from build123d import *

# Parameters (mm, degrees)
SKETCH_R          = 1.45
PAD001_DEPTH      = 1.6
SKETCH001_R       = 1.45
PAD002_DEPTH      = 16.25
POCKET_DEPTH      = 190.001
POCKET_DEPTH_BACK = 0.001
SKETCH003_R       = 1.45
PAD003_DEPTH      = 3.4
POCKET001_DEPTH   = 5
POCKET002_DEPTH   = 10
SKETCH031_R       = 1.125
PAD017_DEPTH      = 6
POCKET013_DEPTH   = 4
SKETCH033_R       = 3
POCKET014_DEPTH   = 5


with BuildPart() as part:
    # Sketch → Pad001 (new body)
    with BuildSketch(Plane.XY):
        with BuildLine():
            Line((12.25, 182), (190.25, 182))
            ThreePointArc((196.25, 176), (194.492641, 180.242641), (190.25, 182))
            Line((196.25, 176), (196.25, 3))
            ThreePointArc((190.25, -3), (194.492641, -1.242641), (196.25, 3))
            Line((190.25, -3), (12.25, -3))
            ThreePointArc((6.25, 3), (8.007359, -1.242641), (12.25, -3))
            Line((6.25, 3), (6.25, 97))
            Line((23.25, 97), (6.25, 97))
            ThreePointArc((23.25, 97), (28.906854, 99.343146), (31.25, 105))
            Line((31.25, 122), (31.25, 105))
            ThreePointArc((31.25, 122), (28.906854, 127.656854), (23.25, 130))
            Line((6.25, 130), (23.25, 130))
            Line((6.25, 130), (6.25, 176))
            ThreePointArc((12.25, 182), (8.007359, 180.242641), (6.25, 176))
        make_face()
        with Locations((11, 173.49762)):
            Circle(SKETCH_R, mode=Mode.SUBTRACT)
        with Locations((11, 89.49762)):
            Circle(SKETCH_R, mode=Mode.SUBTRACT)
        with Locations((180.742493, 173.605331)):
            Circle(SKETCH_R, mode=Mode.SUBTRACT)
        with Locations((181.761108, 91.056091)):
            Circle(SKETCH_R, mode=Mode.SUBTRACT)
        with Locations((44.67, 76.67)):
            Circle(SKETCH_R, mode=Mode.SUBTRACT)
        with Locations((44.67, 24.67)):
            Circle(SKETCH_R, mode=Mode.SUBTRACT)
        with Locations((191.67, 24.67)):
            Circle(SKETCH_R, mode=Mode.SUBTRACT)
        with Locations((191.67, 76.67)):
            Circle(SKETCH_R, mode=Mode.SUBTRACT)
        with BuildLine():
            ThreePointArc((40.25, 97.49762), (42.593146, 91.840766), (48.25, 89.49762))
            Line((168.624548, 89.49762), (48.25, 89.49762))
            ThreePointArc((168.624548, 89.49762), (174.281402, 91.840766), (176.624548, 97.49762))
            Line((176.624548, 122), (176.624548, 97.49762))
            ThreePointArc((176.624548, 122), (174.281402, 127.656854), (168.624548, 130))
            Line((48.25, 130), (168.624548, 130))
            ThreePointArc((48.25, 130), (42.593146, 127.656854), (40.25, 122))
            Line((40.25, 97.49762), (40.25, 122))
        make_face(mode=Mode.SUBTRACT)
        with BuildLine():
            ThreePointArc((15.25, 147), (17.593146, 141.343146), (23.25, 139))
            Line((168.563514, 139), (23.25, 139))
            ThreePointArc((168.563514, 139), (174.220369, 141.343146), (176.563514, 147))
            Line((176.563514, 165.49762), (176.563514, 147))
            ThreePointArc((176.563514, 165.49762), (174.220369, 171.154474), (168.563514, 173.49762))
            Line((23.25, 173.49762), (168.563514, 173.49762))
            ThreePointArc((23.25, 173.49762), (17.593146, 171.154474), (15.25, 165.49762))
            Line((15.25, 147), (15.25, 165.49762))
        make_face(mode=Mode.SUBTRACT)
        with BuildLine():
            ThreePointArc((51.67, 14), (54.013146, 8.343146), (59.67, 6))
            Line((176.67, 6), (59.67, 6))
            ThreePointArc((176.67, 6), (182.326854, 8.343146), (184.67, 14))
            Line((184.67, 68.67), (184.67, 14))
            ThreePointArc((184.67, 68.67), (182.326854, 74.326854), (176.67, 76.67))
            Line((59.67, 76.67), (176.67, 76.67))
            ThreePointArc((59.67, 76.67), (54.013146, 74.326854), (51.67, 68.67))
            Line((51.67, 14), (51.67, 68.67))
        make_face(mode=Mode.SUBTRACT)
    extrude(amount=-PAD001_DEPTH)

    # Sketch001 → Pad002 (join)
    with BuildSketch(Plane.XY):
        with BuildLine():
            ThreePointArc((51.67, 76.67), (44.67, 83.67), (37.67, 76.67))
            Line((37.67, 76.67), (37.67, 7))
            ThreePointArc((37.67, 7), (44.67, 0), (51.67, 7))
            Line((51.67, 7), (51.67, 76.67))
        make_face()
        with Locations((44.67, 76.67)):
            Circle(SKETCH001_R, mode=Mode.SUBTRACT)
        with Locations((44.67, 24.67)):
            Circle(SKETCH001_R, mode=Mode.SUBTRACT)
        with BuildLine():
            ThreePointArc((196.25, 76.67), (191.67, 81.25), (187.09, 76.67))
            Line((187.09, 76.67), (187.09, 4.58))
            ThreePointArc((187.09, 4.58), (191.67, 0), (196.25, 4.58))
            Line((196.25, 4.58), (196.25, 76.67))
        make_face()
        with Locations((191.67, 76.67)):
            Circle(SKETCH001_R, mode=Mode.SUBTRACT)
        with Locations((191.67, 24.67)):
            Circle(SKETCH001_R, mode=Mode.SUBTRACT)
    extrude(amount=PAD002_DEPTH)

    # Sketch002 (on Face56 of Pad002) → Pocket (cut, two sides)
    with BuildSketch(Plane.YZ.offset(196.25)) as pocket_sk:
        with BuildLine():
            ThreePointArc((31, 22), (28.87868, 21.12132), (28, 19))
            Line((28, 9), (28, 19))
            ThreePointArc((28, 9), (28.87868, 6.87868), (31, 6))
            Line((61, 6), (31, 6))
            ThreePointArc((61, 6), (63.12132, 6.87868), (64, 9))
            Line((64, 19), (64, 9))
            ThreePointArc((64, 19), (63.12132, 21.12132), (61, 22))
            Line((31, 22), (61, 22))
        make_face()
    extrude(amount=-POCKET_DEPTH, mode=Mode.SUBTRACT)
    extrude(pocket_sk.sketch, amount=POCKET_DEPTH_BACK, mode=Mode.SUBTRACT)

    # Sketch003 → Pad003 (join)
    with BuildSketch(Plane.XY.offset(-0.1)):
        with BuildLine():
            ThreePointArc((185.53296, 93.654078), (179.163121, 94.827943), (177.989256, 88.458104))
            Line((177.989256, 88.458104), (187.898148, 74.072013))
            ThreePointArc((187.898148, 74.072013), (194.267987, 72.898148), (195.441852, 79.267987))
            Line((195.441852, 79.267987), (185.53296, 93.654078))
        make_face()
        with Locations((191.67, 76.67)):
            Circle(SKETCH003_R, mode=Mode.SUBTRACT)
        with Locations((181.761108, 91.056091)):
            Circle(SKETCH003_R, mode=Mode.SUBTRACT)
        with BuildLine():
            ThreePointArc((12.691088, 93.936395), (6.561225, 91.188708), (9.308912, 85.058845))
            Line((9.308912, 85.058845), (42.978912, 72.231225))
            ThreePointArc((42.978912, 72.231225), (49.108775, 74.978912), (46.361088, 81.108775))
            Line((46.361088, 81.108775), (12.691088, 93.936395))
        make_face()
        with Locations((44.67, 76.67)):
            Circle(SKETCH003_R, mode=Mode.SUBTRACT)
        with Locations((11, 89.49762)):
            Circle(SKETCH003_R, mode=Mode.SUBTRACT)
        with BuildLine():
            ThreePointArc((15.25, 173.49762), (11, 177.74762), (6.75, 173.49762))
            Line((6.75, 173.49762), (6.75, 165.49762))
            ThreePointArc((6.75, 165.49762), (11, 161.24762), (15.25, 165.49762))
            Line((15.25, 165.49762), (15.25, 173.49762))
        make_face()
        with Locations((11, 173.49762)):
            Circle(SKETCH003_R, mode=Mode.SUBTRACT)
        with BuildLine():
            ThreePointArc((180.742493, 178.185331), (176.162493, 173.605331), (180.742493, 169.025331))
            Line((180.742493, 169.025331), (191.67, 169.025331))
            ThreePointArc((191.67, 169.025331), (196.25, 173.605331), (191.67, 178.185331))
            Line((191.67, 178.185331), (180.742493, 178.185331))
        make_face()
        with Locations((180.742493, 173.605331)):
            Circle(SKETCH003_R, mode=Mode.SUBTRACT)
    extrude(amount=PAD003_DEPTH)

    # Sketch004 → Pocket001 (cut)
    with BuildSketch(Plane.XY):
        with BuildLine():
            ThreePointArc((75.723694, 140.85524), (75.016587, 140.562347), (74.723694, 139.85524))
            Line((74.723694, 134.85524), (74.723694, 139.85524))
            ThreePointArc((74.723694, 134.85524), (75.016587, 134.148133), (75.723694, 133.85524))
            Line((91.423694, 133.85524), (75.723694, 133.85524))
            ThreePointArc((91.423694, 133.85524), (92.130801, 134.148133), (92.423694, 134.85524))
            Line((92.423694, 139.85524), (92.423694, 134.85524))
            ThreePointArc((92.423694, 139.85524), (92.130801, 140.562347), (91.423694, 140.85524))
            Line((75.723694, 140.85524), (91.423694, 140.85524))
        make_face()
        with BuildLine():
            ThreePointArc((129.923694, 140.85524), (129.216587, 140.562347), (128.923694, 139.85524))
            Line((128.923694, 134.85524), (128.923694, 139.85524))
            ThreePointArc((128.923694, 134.85524), (129.216587, 134.148133), (129.923694, 133.85524))
            Line((145.623694, 133.85524), (129.923694, 133.85524))
            ThreePointArc((145.623694, 133.85524), (146.330801, 134.148133), (146.623694, 134.85524))
            Line((146.623694, 139.85524), (146.623694, 134.85524))
            ThreePointArc((146.623694, 139.85524), (146.330801, 140.562347), (145.623694, 140.85524))
            Line((129.923694, 140.85524), (145.623694, 140.85524))
        make_face()
    extrude(amount=-POCKET001_DEPTH, mode=Mode.SUBTRACT)

    # Sketch008 → Pocket002 (cut, symmetric)
    with BuildSketch(Plane.XY):
        with BuildLine():
            Line((26.73, 3), (26.73, 85.058845))
            Line((26.73, 85.058845), (-23.27, 85.058845))
            Line((-23.27, 85.058845), (-23.27, -53))
            Line((-23.27, -53), (32.73, -53))
            Line((32.73, -53), (32.73, -3))
            ThreePointArc((26.73, 3), (28.487359, -1.242641), (32.73, -3))
        make_face()
    extrude(amount=POCKET002_DEPTH, both=True, mode=Mode.SUBTRACT)

    # Sketch031 → Pad017 (join)
    with BuildSketch(Plane.XZ.offset(-6)):
        with BuildLine():
            Line((44.67, 0), (191.67, 0))
            Line((191.67, 0), (191.67, 13))
            Line((191.67, 13), (148.458463, 13))
            Line((148.458463, 13), (148.458463, 40.730738))
            ThreePointArc((148.458463, 40.730738), (147.491915, 43.06419), (145.158463, 44.030738))
            Line((145.158463, 44.030738), (67.158463, 44.030738))
            ThreePointArc((67.158463, 44.030738), (64.825011, 43.06419), (63.858463, 40.730738))
            Line((63.858463, 40.730738), (63.858463, 13))
            Line((63.858463, 13), (44.67, 13))
            Line((44.67, 13), (44.67, 0))
        make_face()
        with Locations((67.158463, 40.730738)):
            Circle(SKETCH031_R, mode=Mode.SUBTRACT)
        with Locations((67.158463, 6.980738)):
            Circle(SKETCH031_R, mode=Mode.SUBTRACT)
        with Locations((145.158463, 40.730738)):
            Circle(SKETCH031_R, mode=Mode.SUBTRACT)
        with Locations((145.158463, 6.980738)):
            Circle(SKETCH031_R, mode=Mode.SUBTRACT)
    extrude(amount=PAD017_DEPTH)

    # Sketch032 (on Face13 of Pad017) → Pocket013 (cut)
    with BuildSketch(Plane(origin=(0, 6, 0), x_dir=(-1, 0, 0), z_dir=(0, 1, 0))):
        with BuildLine():
            Line((-64.858463, 37.430738), (-64.858463, 13.030738))
            Line((-64.858463, 13.030738), (-95.458463, 13.030738))
            Line((-95.458463, 13.030738), (-95.458463, 43.030738))
            Line((-95.458463, 43.030738), (-70.458463, 43.030738))
            Line((-70.458463, 43.030738), (-70.458463, 40.730738))
            ThreePointArc((-70.458463, 40.730738), (-69.491914, 38.397285), (-67.158461, 37.430738))
            Line((-67.158461, 37.430738), (-64.858463, 37.430738))
        make_face()
    extrude(amount=-POCKET013_DEPTH, mode=Mode.SUBTRACT)

    # Sketch033 (on Face113 of Pocket013) → Pocket014 (cut)
    with BuildSketch(Plane.XY.offset(16.25)):
        with Locations((51.67, 74.25)):
            Circle(SKETCH033_R)
    extrude(amount=-POCKET014_DEPTH, mode=Mode.SUBTRACT)


with BuildPart() as part_1:
    # Body001 placement: moved
    add(part.part.moved(Location((0, 0, -3.4))))


solid = part_1.part
Model file for the job. Use its own axes, mm. A direction names the side the tool comes from. Coordinates: 2 decimals unless noted, no trailing zeros. Write each loop counter-clockwise with the first axis right and the second up, starting at its lowest first coordinate (ties: lowest second). Pieces come first, ordered by that corner, then holes. Notation, with made-up numbers: (55, 43.25) - (66, 43.25) arc R15 cw to (66, 61.25) - close; hole circle Ø9 at (6.25, 86). An arc over 180 degrees is marked (long way). Write each question's results on one line, items separated by ' | '. Start each with the question number.
1) Flat gauge pins, fed straight in: P1, Ø3.5, axis at x = 193.5, z = 10.5, coming from the +Y side; P2, Ø1.5, axis at x = 15, z = -2.5, coming from the -Y side; P3, Ø5, axis at x = 76.5, z = 7, coming from the -Y side. Where does each tip first touch, or does it go through?
2) 3-axis set-ups, long thin cutter, end or side, ignore diameter. For faces 1 (the face through (26.73, 53, -4)), 2 (the face through (174.282, 171.092, -4.189)), 3 (the face through (45, 46, 2.6)), 4 (the face through (28.844, 99.281, -4.189)), 5 (the face through (10.91, 161.25, -1.77)): which of +Z, -Z, +X, -X, +Y, -Y reach the whole face in a straight line?
3) Cut at B-B (x = 152.5). Write the cut outline in (y, z).
4) Cut at C-C (z = 22). Write the cut outline in (x, y).
5) Cut at D-D (y = 20). Write the cut outline in (x, z).
6) Mould opens along Y. For faces 6 (the face through (184, 88, -0.1)), 7 (the face through (192, 28, 9)), 8 (the face through (11.093, 177.747, -1.773)) say: pulls with the +Y half, pulls with the -Y half, needs draft (parallel to the pull), parting line crosses it, or undercut.
7) Probe line 1 along Y through (x, z) = (11, -3); line 2 along X through (y, z) = (68, 9.5); line 3 along Y through (x, z) = (170.5, -1.5). List the from-to ranges inside material, lowest first. Write a range as from..to.
8) Cut at A-A (y = 43). Write the cut outline in (x, z).
Returned:
1) P1: y = 81.25 | P2: y = 85.06 | P3: y = 0
2) face 1: +Z, -Z, -X, -Y | face 2: +Z, -Z | face 3: +Z, +X, -X | face 4: +Z, -Z, -X | face 5: +Z
3) outline: (-3, -5) - (6, -5) - (6, 9.6) - (0, 9.6) - (0, -3.4) - (-3, -3.4) - close; (76.67, -5) - (89.5, -5) - (89.5, -3.4) - (76.67, -3.4) - close; (130, -5) - (139, -5) - (139, -3.4) - (130, -3.4) - close; (173.5, -5) - (182, -5) - (182, -3.4) - (173.5, -3.4) - close
4) outline: (63.86, 0) - (148.46, 0) - (148.46, 6) - (95.46, 6) - (95.46, 2) - (64.86, 2) - (64.86, 6) - (63.86, 6) - close
5) outline: (26.73, -5) - (51.67, -5) - (51.67, 12.85) - (37.67, 12.85) - (37.67, -3.4) - (26.73, -3.4) - close; (184.67, -5) - (196.25, -5) - (196.25, 12.85) - (187.09, 12.85) - (187.09, -3.4) - (184.67, -3.4) - close
6) face 6: needs draft | face 7: undercut | face 8: pulls with the +Y half
7) line 1: 85.06..88.05, 90.95..94.25, 161.25..172.05, 174.95..177.75 | line 2: 37.67..51.67, 187.09..196.25 | line 3: 0..6
8) outline: (26.73, -5) - (51.67, -5) - (51.67, 2.6) - (37.67, 2.6) - (37.67, -3.4) - (26.73, -3.4) - close; (184.67, -5) - (196.25, -5) - (196.25, 2.6) - (187.09, 2.6) - (187.09, -3.4) - (184.67, -3.4) - close
